Answer from the drawing. Dimensions are ordinates in mm from the lowest x, y and z of the part. A direction names the side the tool comes from. Coordinates: 2 decimals unless noted, no trailing zeros. Write each loop counter-clockwise with the first axis right and the second up, starting at its lowest first coordinate (ties: lowest second). Pieces come first, ordered by that corner, then holes. Notation, with made-up numbers: (46, -23.75) -> (80, -23.75) arc R25 ccw to (80, 7.25) -> close; hole circle Ø6 at (-16, -19.75). An arc over 180 degrees is marked (long way). Return JSON: item names as keys, results as strings.
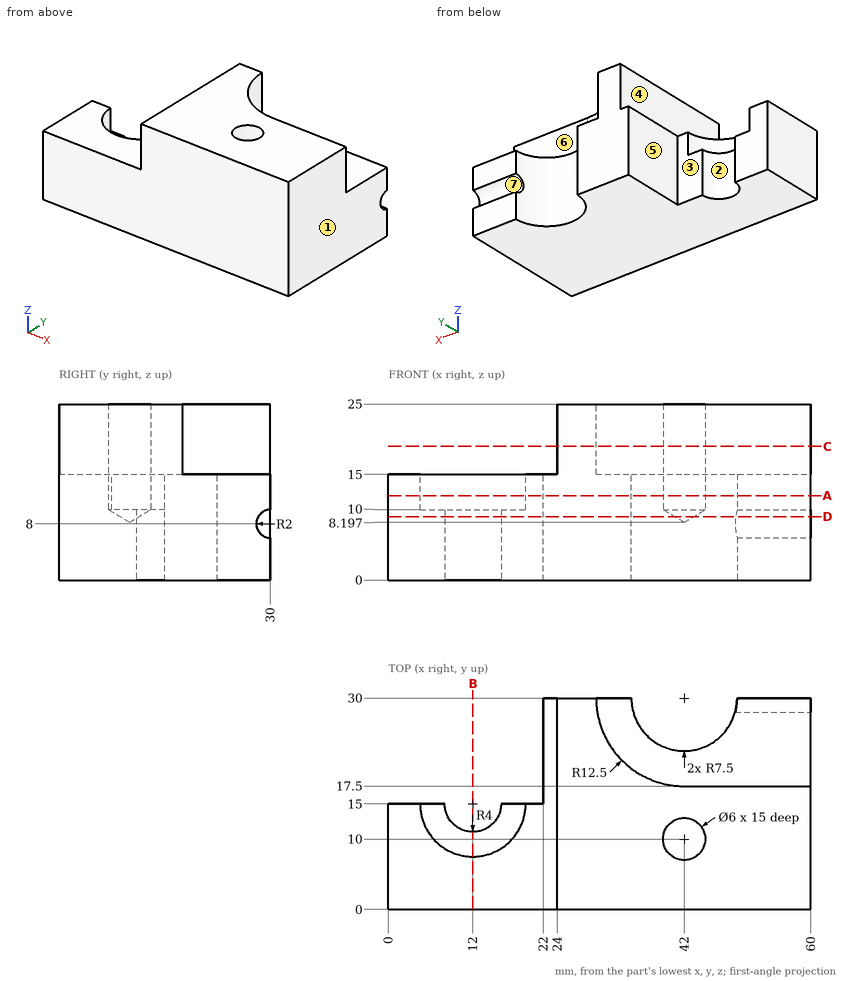
1. Consider L1, parallel to Y at x = 42, z = 15.5; L2, parallel to Y at x = 42, z = 13.75; L3, parallel to X at y = 10, z = 18. Determine where each line is inside the solid, lowest interval first.
Taken from the geometry:
{"L1": "y = 0 to 7, 13 to 17.5", "L2": "y = 0 to 7, 13 to 22.5", "L3": "x = 24 to 39, 45 to 60"}
2. Flat-ended cylindrical pins translate along their axes: pin 1 Ø10 at (y, z) = (14.5, 20.5) entering from -X; pin 2 Ø2.5 at (x, z) = (2.5, 8.5) entering from +Y; pin 3 Ø6 at (x, y) = (11, 11) entering from +Z. Find the tip coordinate at first contact, or state that the pin passes through.
Taken from the geometry:
{"pin 1": "stops at x = 24", "pin 2": "stops at y = 15", "pin 3": "stops at z = 10"}
3. The part is cut by section B-B (x = 12). Determine the outline of the cut face in (y, z).
Taken from the geometry:
{"outline": "(0, 0) -> (11, 0) -> (11, 10) -> (7.5, 10) -> (7.5, 15) -> (0, 15) -> close"}
4. A tool of negligible diameter and unlimited length cuts with its end or side. For the marked faces 5, 6 and 7, from which of +Z, -Z, +X, -X, +Y, -Y can it reach the whole face along a straight path? Write none if from no direction.
Taken from the geometry:
{"face 5": "+Z, -Z, -X, +Y", "face 6": "+Z, +X, +Y", "face 7": "+X, +Y"}
5. The part is cut by section D-D (z = 9). Determine the outline of the cut face in (x, y) (1 decimal), then the cut area to 3 significant figures.
Taken from the geometry:
{"outline": "(0, 0) -> (60, 0) -> (60, 28.3) -> (49.3, 28.3) arc R7.5 cw to (34.5, 30) -> (22, 30) -> (22, 15) -> (16, 15) arc R4 cw to (8, 15) -> (0, 15) -> close; hole circle Ø2.7 at (42, 10)", "area": "1,330 mm2"}
6. The part is cut by section C-C (z = 19). Determine the outline of the cut face in (x, y), then the cut area to 3 significant figures.
Taken from the geometry:
{"outline": "(24, 0) -> (60, 0) -> (60, 17.5) -> (42, 17.5) arc R12.5 cw to (29.5, 30) -> (24, 30) -> close; hole circle Ø6 at (42, 10)", "area": "704 mm2"}
7. The part is cut by section A-A (z = 12). Determine the outline of the cut face in (x, y).
Taken from the geometry:
{"outline": "(0, 0) -> (60, 0) -> (60, 30) -> (49.5, 30) arc R7.5 cw to (34.5, 30) -> (22, 30) -> (22, 15) -> (19.5, 15) arc R7.5 cw to (4.5, 15) -> (0, 15) -> close; hole circle Ø6 at (42, 10)"}
8. For a pull along X with two mould halves and no side action, classify the marked faces 1, 2, 3 and 4 as +X half, -X half, draft (parallel to the pull), parting line (faces both ways), or undercut.
Taken from the geometry:
{"face 1": "+X half", "face 2": "undercut", "face 3": "draft", "face 4": "-X half"}
